from build123d import *

# Parameters (mm, degrees)
SKETCH_1_W          = 20
SKETCH_1_H          = 20
EXTRUDE_1_DEPTH     = 10
SKETCH_1_3_W        = 5
SKETCH_1_3_H        = 10
SKETCH_1_3_W_2      = 10
EXTRUDE_2_DEPTH     = 20
SKETCH_2_W          = 5
SKETCH_2_H          = 5
CUT_EXTRUDE_1_DEPTH = 20
FILLET_1_R          = 10


with BuildPart() as part:
    # Sketch 1 → Extrude 1 (new body)
    with BuildSketch(Plane(origin=(0, 0, 0), x_dir=(1, 0, 0), z_dir=(0, 1, 0))):
        Rectangle(SKETCH_1_W, SKETCH_1_H)
        Polygon((-5, 5), (-5, -5), (5, 5), align=None, mode=Mode.SUBTRACT)
    extrude(amount=EXTRUDE_1_DEPTH)

    # Sketch 1_3 → Extrude 2 (add)
    with BuildSketch(Plane(origin=(0, 0, 0), x_dir=(1, 0, 0), z_dir=(0, 1, 0))):
        with Locations((-7.5, 15)):
            Rectangle(SKETCH_1_3_W, SKETCH_1_3_H)
        with Locations((0, 15)):
            Rectangle(SKETCH_1_3_W_2, SKETCH_1_3_H)
        with Locations((7.5, 15)):
            Rectangle(SKETCH_1_3_W, SKETCH_1_3_H)
    extrude(amount=EXTRUDE_2_DEPTH)

    # Sketch 2 → Cut-Extrude 1 (cut)
    with BuildSketch(Plane.XY.offset(-10)):
        Polygon((5, 20), (-5, 20), (5, 15), align=None)
        with Locations((7.5, 17.5)):
            Rectangle(SKETCH_2_W, SKETCH_2_H)
    extrude(amount=-CUT_EXTRUDE_1_DEPTH, mode=Mode.SUBTRACT)

    # Fillet 1
    fillet_1_edges = [part.edges().sort_by_distance(p)[0] for p in [
        (10, 5, 10),
    ]]
    fillet(fillet_1_edges, radius=FILLET_1_R)


solid = part.part
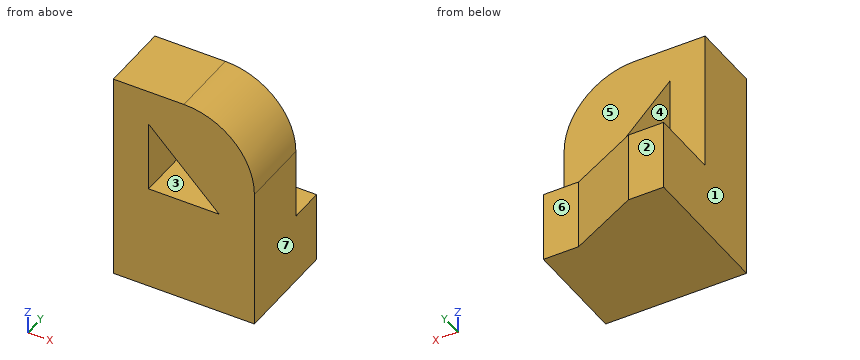
Geometry check sheet. Reference: the model listing, model coordinates, mm. Face numbers are marked on the shaded views. A direction names the side the tool comes from. Round coordinates to 2 decimals unless told otherwise and drop trailing zeros. Loops run counter-clockwise (first coordinate to the right, second up) from the corner with the lowest first, then second, coordinate; pieces in that order, holes last. Notation, with made-up numbers: (25, -17) -> (74, -17) arc R19 ccw to (74, 18) -> close; hole circle Ø6 at (-28, 20.25). An arc over 180 degrees is marked (long way). Answer as a JSON object with one key per item and string values. Group by question number.
Item 1: Cross-section at C-C, the plane y = 1.5. Record the cut outline in (x, z).
Item 2: Thickness scan on line 1 along Y through (x, z) = (-3.5, -5.5); line 2 along Z through (x, y) = (-7, 18.25); line 3 along Z through (x, y) = (4, 9.5). Record the ranges inside material, lowest first.
Item 3: Depth check by flat-ended pin: pin 1 Ø2.5 at (x, z) = (8, -12.5) entering from +Y; pin 2 Ø3 at (x, z) = (-1, 0.5) entering from +Y; pin 3 Ø5 at (x, y) = (4.5, 7) entering from +Z. Enter the tip coordinate at first touch or a pass-through.
Item 4: Release check for a two-part mould opening along X. For the marked faces 1, 2 and 3 record: pulls with the +X half, pulls with the -X half, needs draft (parallel to the pull), parting line crosses it, or undercut.
Item 5: Set-up check for the marked faces 4, 5, 6 and 7: record each of +Z, -Z, +X, -X, +Y, -Y from which the full face is reachable in a straight line by a thin tool's end or side.
Item 6: Cross-section at B-B, the plane z = -2.25. Record the cut outline in (x, y), plus the area to 4 significant figures.
Item 7: Cross-section at A-A, the plane x = -2. Record the cut outline in (y, z).
Item 8: Cross-section at D-D, the plane x = 8. Record the cut outline in (y, z).
Determined:
{
 "1": {"outline": "(-10, -20) -> (10, -20) -> (10, 0) arc R10 ccw to (0, 10) -> (-10, 10) -> close; hole (-5, -5) -> (5, -5) -> (-5, 5) -> close"},
 "2": {"line 1": "y = 0 to 10", "line 2": "z = -20 to -10", "line 3": "z = -20 to -5, -4 to 9.17"},
 "3": {"pin 1": "stops at y = 15", "pin 2": "stops at y = 10", "pin 3": "stops at z = 9.8"},
 "4": {"face 1": "pulls with the -X half", "face 2": "needs draft", "face 3": "undercut"},
 "5": {"face 4": "+Y, -Y", "face 5": "+Z, +X, -X, +Y", "face 6": "+Z, -Z, +X, +Y", "face 7": "+Z, -Z, +X, +Y, -Y"},
 "6": {"outline": "(-10, 0) -> (-5, 0) -> (-5, 10) -> (-10, 10) -> close; (2.25, 0) -> (10, 0) -> (10, 10) -> (2.25, 10) -> close", "area": "127.5 mm²"},
 "7": {"outline": "(0, -20) -> (18.5, -20) -> (18.5, -10) -> (10, -10) -> (10, -5) -> (0, -5) -> close; (0, 2) -> (10, 2) -> (10, 10) -> (0, 10) -> close"},
 "8": {"outline": "(0, -20) -> (15, -20) -> (15, -10) -> (10, -10) -> (10, 6) -> (0, 6) -> close"}
}
